Part model, mm, in its own coordinate system. Face numbers are marked on the shaded views. A direction names the side the tool comes from. Round coordinates to 2 decimals unless told otherwise and drop trailing zeros. Write each loop counter-clockwise with the first axis right and the second up, starting at its lowest first coordinate (ties: lowest second). Pieces come first, ordered by that corner, then holes. Notation, with made-up numbers: M 67.5,-22.5 L 100.5,-22.5 A11 ccw 100.5,-10.5 Z; hole C -16,6.25 d11. An arc over 180 degrees is marked long. Answer as a JSON object with one key per item and string values. Group by question number.
1. Band-saw the part on C-C, the plane x = 30. Write the cut outline in (y, z), plus the area to 3 significant figures.
2. Drop flat-ended pins along their axis: pin 1 (13 mm diameter, centred on x = 22.94, z = 13.97, fed in from -Y); pin 2 (23 mm diameter, centred on x = -9.5, y = 4.5, fed in from +Z); pin 3 (12 mm diameter, centred on x = 8.5, y = -4, fed in from -Z). Give the stop position or say it passes through.
3. Which spindle directions (+Z, -Z, +X, -X, +Y, -Y) get a long thin tool onto all of the face, cutting with end or side? Do the marked faces 5 and 6. Say none if no direction does.
4. Band-saw the part on B-B, the plane x = 9.5. Write the cut outline in (y, z).
5. Drill centre lines: line 1 (X direction, y = -24.05, z = 13.97); line 2 (Y direction, x = -25, z = 6); line 3 (X direction, y = -15.5, z = 17.5). Where is each one in solid material? Low to high. Write a range as from..to.
6. Band-saw the part on A-A, the plane y = -3.5. Write the cut outline in (x, z).
7. Two-plate mould, pull along X, no slides. Class the marked faces 1, 2, 3 and 4: +X half, -X half, draft (parallel to the pull), parting line (faces both ways), or undercut.
8. Band-saw the part on D-D, the plane z = 20.75. Write the cut outline in (x, y), plus the area to 3 significant figures.
from build123d import *

# Parameters (mm, degrees)
F0_W      = 76.2
F0_H      = 50.8
F1_DEPTH  = 2.54
F3_DEPTH  = 22.86
F5_DEPTH  = 25.4
F7_DEPTH  = 25.4
F8_W      = 4.318
F8_H      = 7.62
F9_DEPTH  = 25.4
F10_W     = 5.08
F10_H     = 2.54
F11_DEPTH = 25.4
F12_SIZE  = 1.27


with BuildPart() as f1:
    # F0 (on Top) → F1 (new body)
    with BuildSketch(Plane.XY):
        with Locations((5.156827, 0.141645)):
            Rectangle(F0_W, F0_H)
    extrude(amount=F1_DEPTH)

    # F2 (on face) → F3 (join)
    with BuildSketch(Plane.XY.offset(2.54)):
        Polygon((-30.403173, -22.718355), (-30.403173, 23.001645), (40.716827, 23.001645), (40.716827, -5.898658), (43.256827, -5.898658), (43.256827, 25.541645), (-32.943173, 25.541645), (-32.943173, -25.258355), (19.057203, -25.258355), (19.057203, -22.718355), align=None)
        Polygon((43.256827, -5.898658), (40.716827, -5.898658), (40.716827, -22.718355), (19.057203, -22.718355), (19.057203, -25.258355), (43.256827, -25.258355), align=None)
    extrude(amount=F3_DEPTH)

    # F4 (on face) → F5 (cut)
    with BuildSketch(Plane.XZ.offset(25.258355)):
        with BuildLine():
            Line((22.936827, 13.97), (31.191827, 13.97))
            ThreePointArc((31.191827, 13.97), (17.09966, 19.807166), (22.936827, 5.715))
            Line((22.936827, 5.715), (22.936827, 13.97))
        make_face()
        with BuildLine():
            ThreePointArc((22.936827, 5.715), (28.773993, 8.132834), (31.191827, 13.97))
            Line((31.191827, 13.97), (22.936827, 13.97))
            Line((22.936827, 13.97), (22.936827, 5.715))
        make_face()
    extrude(amount=-F5_DEPTH, mode=Mode.SUBTRACT)

    # F6 (on face) → F7 (cut)
    with BuildSketch(Plane.YZ.offset(43.256827)):
        with BuildLine():
            ThreePointArc((-11.288355, 9.398), (-8.055463, 10.737108), (-6.716355, 13.97))
            ThreePointArc((-6.716355, 13.97), (-11.288355, 18.542), (-15.860355, 13.97))
            Line((-15.860355, 13.97), (-11.288355, 13.97))
            Line((-11.288355, 13.97), (-11.288355, 9.398))
        make_face()
        with BuildLine():
            Line((-11.288355, 13.97), (-15.860355, 13.97))
            ThreePointArc((-15.860355, 13.97), (-14.521247, 10.737108), (-11.288355, 9.398))
            Line((-11.288355, 9.398), (-11.288355, 13.97))
        make_face()
    extrude(amount=-F7_DEPTH, mode=Mode.SUBTRACT)

    # F8 (on face) → F9 (cut)
    with BuildSketch(Plane.XZ.offset(25.258355)):
        with Locations((-28.244173, 12.7)):
            Rectangle(F8_W, F8_H)
    extrude(amount=-F9_DEPTH, mode=Mode.SUBTRACT)

    # F10 (on face) → F11 (cut)
    with BuildSketch(Plane(origin=(-32.943173, 0, 0), x_dir=(0, -1, 0), z_dir=(-1, 0, 0))):
        with Locations((4.938355, 3.81)):
            Rectangle(F10_W, F10_H)
    extrude(amount=-F11_DEPTH, mode=Mode.SUBTRACT)

    # F12
    f12_edges = [f1.edges().sort_by_distance(p)[0] for p in [
        (5.156827, 23.001645, 25.4),
        (-30.403173, 0.141645, 25.4),
        (40.716827, 0.141645, 25.4),
        (5.156827, -22.718355, 25.4),
    ]]
    chamfer(f12_edges, length=F12_SIZE)


solid = f1.part
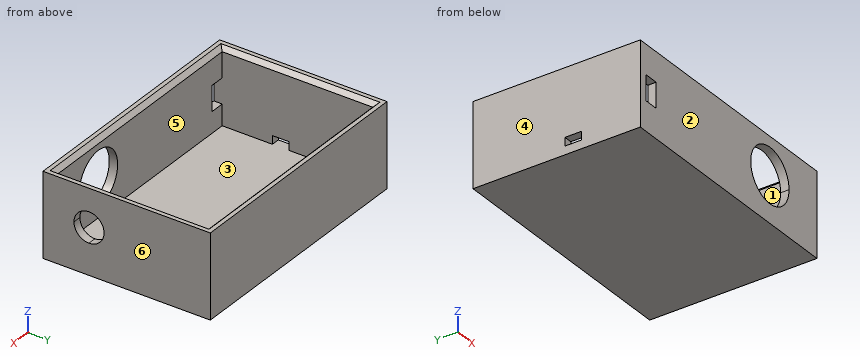
Worked answers:
{
 "1": {"outline": "M -25.26,0 L 25.54,0 L 25.54,25.4 L 24.27,25.4 L 23,24.13 L 23,2.54 L -22.72,2.54 L -22.72,9.7 L -25.26,9.7 Z; M -25.26,18.24 L -22.72,18.24 L -22.72,24.13 L -23.99,25.4 L -25.26,25.4 Z", "area": "222 mm^2"},
 "2": {"pin 1": "stops at y = 23", "pin 2": "stops at z = 2.54", "pin 3": "stops at z = 0"},
 "3": {"face 5": "+Z", "face 6": "+Z, -Z, +X, +Y, -Y"},
 "4": {"outline": "M -25.26,0 L 25.54,0 L 25.54,25.4 L 24.27,25.4 L 23,24.13 L 23,2.54 L -22.72,2.54 L -22.72,24.13 L -23.99,25.4 L -25.26,25.4 Z"},
 "5": {"line 1": "x = -32.94..-30.4, -26.09..14.68, 31.19..43.26", "line 2": "y = -25.26..-22.72, 23..25.54", "line 3": "x = -32.94..-30.4, 40.72..43.26"},
 "6": {"outline": "M -32.94,0 L 43.26,0 L 43.26,25.4 L 41.99,25.4 L 40.72,24.13 L 40.72,2.54 L -32.94,2.54 Z; M -32.94,5.08 L -30.4,5.08 L -30.4,24.13 L -31.67,25.4 L -32.94,25.4 Z"},
 "7": {"face 1": "undercut", "face 2": "draft", "face 3": "undercut", "face 4": "-X half"},
 "8": {"outline": "M -32.94,-25.26 L 18.23,-25.26 L 18.23,-22.72 L -30.4,-22.72 L -30.4,23 L 40.72,23 L 40.72,-22.72 L 27.65,-22.72 L 27.65,-25.26 L 43.26,-25.26 L 43.26,25.54 L -32.94,25.54 Z", "area": "595 mm^2"}
}
